from build123d import *

# Parameters (mm, degrees)
SKETCH_1_R          = 6.25
SKETCH_1_R_2        = 1.25
EXTRUDE_1_DEPTH     = 5
EXTRUDE_START       = 5
SKETCH_1_5_R        = 6.25
EXTRUDE_2_DEPTH     = 1
SKETCH_2_R          = 4.5
EXTRUDE_3_DEPTH     = 7.4
CUT_EXTRUDE_START   = 7.4
CUT_EXTRUDE_1_DEPTH = 7.4
FILLET_1_R          = 0.2


with BuildPart() as part:
    # 草图1 → 凸台-拉伸1 (new body)
    with BuildSketch(Plane.XY):
        Circle(SKETCH_1_R)
        Circle(SKETCH_1_R_2, mode=Mode.SUBTRACT)
    extrude(amount=EXTRUDE_1_DEPTH)

    # 草图1<5> → 凸台-拉伸2 (add)
    with BuildSketch(Plane.XY.offset(EXTRUDE_START)):
        Circle(SKETCH_1_5_R)
    extrude(amount=EXTRUDE_2_DEPTH)

    # 草图2 → 凸台-拉伸3 (add)
    with BuildSketch(Plane.XY.offset(6)):
        Circle(SKETCH_2_R)
    extrude(amount=EXTRUDE_3_DEPTH)

    # 草图2<3> → 切除-拉伸1 (cut)
    with BuildSketch(Plane.XY.offset(6).offset(CUT_EXTRUDE_START)):
        with BuildLine():
            Line((-1.130029762, -1.130029762), (-1.130029762, -2.230029762))
            ThreePointArc((-1.130029762, -2.230029762), (0, -2.5), (1.130029762, -2.230029762))
            Line((1.130029762, -2.230029762), (1.130029762, -1.130029762))
            Line((1.130029762, -1.130029762), (2.230029762, -1.130029762))
            ThreePointArc((2.230029762, -1.130029762), (2.5, 0), (2.230029762, 1.130029762))
            Line((2.230029762, 1.130029762), (1.130029762, 1.130029762))
            Line((1.130029762, 1.130029762), (1.130029762, 2.230029762))
            ThreePointArc((1.130029762, 2.230029762), (0, 2.5), (-1.130029762, 2.230029762))
            Line((-1.130029762, 2.230029762), (-1.130029762, 1.130029762))
            Line((-1.130029762, 1.130029762), (-2.230029762, 1.130029762))
            ThreePointArc((-2.230029762, 1.130029762), (-2.5, 0), (-2.230029762, -1.130029762))
            Line((-2.230029762, -1.130029762), (-1.130029762, -1.130029762))
        make_face()
    extrude(amount=-CUT_EXTRUDE_1_DEPTH, mode=Mode.SUBTRACT)

    # 圆角1
    fillet_1_edges = [part.edges().sort_by_distance(p)[0] for p in [
        (-1.130029762, -1.130029762, 9.7),
        (-1.130029762, 1.130029762, 9.7),
        (1.130029762, 1.130029762, 9.7),
        (1.130029762, -1.130029762, 9.7),
    ]]
    fillet(fillet_1_edges, radius=FILLET_1_R)


solid = part.part
Here's how the part is built. I have some questions about the finished solid (model axes, mm). A direction names the side the tool comes from. Coordinates: 2 decimals unless noted, no trailing zeros. Order: outer loops, then holes, each group sorted by start corner. A loop starts at its lowest first (then second) coordinate and runs counter-clockwise, first axis right, second up.
Item 1: I need wall thicknesses on line 1 (Y direction, x = 0, z = 3.4); line 2 (Z direction, x = 2.25, y = 5.25); line 3 (Y direction, x = 3.5, z = 7). Which ranges of each line are inside material? Lowest first, please.
Result sheet:
line 1: y = -6.25 to -1.25, 1.25 to 6.25
line 2: z = 0 to 6
line 3: y = -2.83 to 2.83
Item 2: For P1, Ø0.5, axis at x = -2, z = 9, coming from the -Y side; P2, Ø0.7, axis at y = 2, z = 8.5, coming from the -X side; P3, Ø1, axis at x = -1.5, z = 8.5, coming from the +Y side, each with a flat end and sliding along its axis, tell me the tip position at first contact or that it passes through.
Result sheet:
P1: stops at y = -4.15
P2: stops at x = -4.19
P3: stops at y = 4.39
Item 3: If we section it at B-B on x = 0: List the corners of the cut face in (y, z) for me, plus the area to 3 significant figures.
Result sheet:
outline: (-6.25, 0) - (-1.25, 0) - (-1.25, 5) - (1.25, 5) - (1.25, 0) - (6.25, 0) - (6.25, 6) - (4.5, 6) - (4.5, 13.4) - (2.5, 13.4) - (2.5, 6) - (-2.5, 6) - (-2.5, 13.4) - (-4.5, 13.4) - (-4.5, 6) - (-6.25, 6) - close
area: 92.1 mm2
Item 4: If we section it at A-A on z = 11.75: List the corners of the cut face in (x, y) for me, plus the area to 3 significant figures.
Result sheet:
outline: circle Ø9 at (0, 0); hole (-2.23, -1.13) - (-1.33, -1.13) arc R0.2 cw to (-1.13, -1.33) - (-1.13, -2.23) arc R2.5 ccw to (1.13, -2.23) - (1.13, -1.33) arc R0.2 cw to (1.33, -1.13) - (2.23, -1.13) arc R2.5 ccw to (2.23, 1.13) - (1.33, 1.13) arc R0.2 cw to (1.13, 1.33) - (1.13, 2.23) arc R2.5 ccw to (-1.13, 2.23) - (-1.13, 1.33) arc R0.2 cw to (-1.33, 1.13) - (-2.23, 1.13) arc R2.5 ccw to start
area: 46.9 mm2
Item 5: If we mould it in two halves opening along X, with no side actions, what happens to faces 1 (the face through (0, -2.5, 9.8)), 2 (the face through (5.96, 1.88, 2.96)), 3 (the face through (3, -4, 6))? For each: +X half, -X half, draft (parallel to the pull), parting line (faces both ways), or undercut.
Result sheet:
face 1: undercut
face 2: parting line
face 3: draft
Item 6: For faces 4 (the face through (-0.1, 1.5, 0)), 5 (the face through (-1.13, -2, 10)), 6 (the face through (0, 0, 5)), which set-ups out of +Z, -Z, +X, -X, +Y, -Y let a thin tool reach every point of the face, with its end or its side?
Result sheet:
face 4: -Z, +X, -X, +Y, -Y
face 5: +Z
face 6: -Z
Item 7: If we section it at D-D on z = 5.75: List the corners of the cut face in (x, y) for me, plus the area to 3 significant figures.
Result sheet:
outline: circle Ø12.5 at (0, 0)
area: 123 mm2
